Can you work these out from the model? Positions are in its coordinate system, mm. Give positions to 0.01 mm unless a question says otherwise; leave off trailing zeros. Write each loop counter-clockwise with the first axis right and the second up, starting at its lowest first coordinate (ties: lowest second). Pieces come first, ordered by that corner, then holes.
1. Suppose I cut it at C-C (z = 28). Please give me the cut outline in (x, y), and give its area (3 significant figures).
2. Suppose I cut it at D-D (y = -25). Please give me the cut outline in (x, z).
3. Suppose I cut it at B-B (x = 6). Please give me the cut outline in (y, z), and give its area (3 significant figures).
4. Suppose I cut it at A-A (y = 0). Please give me the cut outline in (x, z), and give its area (3 significant figures).
5. I'm going to push a flat-ended pin straight in: pin 1 (5 mm diameter, centred on x = 6, y = 25, fed in from -Z). Where does the tip first touch, or does it pass through?
6. If I drill on probe 1 along Y at (x, z) = (5.25, -16), over which ranges is the centre line in solid material (lowest first)?
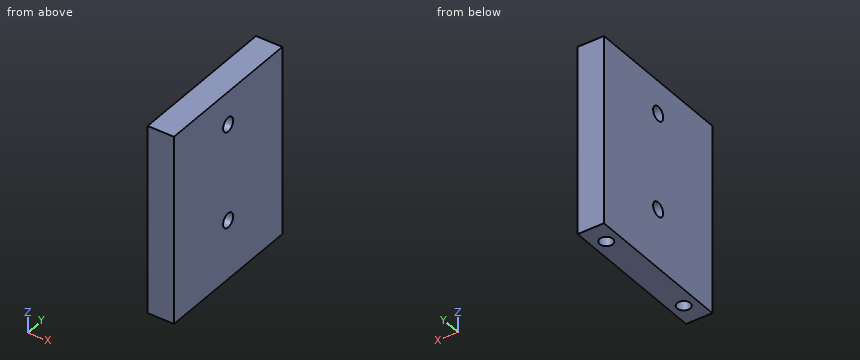
Autodesk Inventor part; units mm, degrees
ref_plane "YZ Plane" through (0, 0, 0) normal (1, 0, 0) x (0, 1, 0)
ref_plane "XZ Plane" through (0, 0, 0) normal (0, 1, 0) x (-1, 0, 0)
ref_plane "XY Plane" through (0, 0, 0) normal (0, 0, 1) x (1, 0, 0)
sketch "Sketch1" plane through (0, 0, 0) normal (1, 0, 0) x (0, 1, 0)
  line L0 (-35, 43) -> (35, 43)
  line L1 (35, 43) -> (35, -43)
  line L2 (35, -43) -> (-35, -43)
  line L3 (-35, -43) -> (-35, 43)
  line L4 (-35, 43) -> (35, -43) construction
  line L5 (35, 43) -> (-35, -43) construction
  point P0 (0, 0)
  dimension "d0" = 86
  dimension "d1" = 70
extrude "Extrusion1" add sketch "Sketch1" along normal blind 12
ref_plane "Work Plane1" through (0, 0, 43) normal (0, 1, 0) x (1, 0, 0)
sketch "Sketch2" plane through (0, -35, -43) normal (0, 0, -1) x (-1, 0, 0)
  circle A0 centre (-6, 60) radius 3
  circle A1 centre (-6, 35) radius 3 construction
  circle A2 centre (-6, 10) radius 3
  line L0 (0, 70) -> (-12, 70)
  line L1 (-6, 70) -> (-6, 0) construction
  line L2 (0, 0) -> (-12, 0)
  point P0 (0, 35)
  dimension "d4" = 6
  dimension "d5" = 25
  dimension "d6" = 25
extrude "Extrusion2" cut sketch "Sketch2" against normal blind 15
sketch "Sketch3" plane through (12, 0, 0) normal (1, 0, 0) x (0, 0, -1)
  circle A0 centre (-46.1752, 0) radius 3
  circle A1 centre (-111.1482, 0) radius 3
  circle A2 centre (-90.1752, 0) radius 3
  point P0 (0, 0)
extrude "Extrusion3" cut sketch "Sketch3" against normal through all
sketch "Sketch4" plane through (0, 0, 0) normal (-1, 0, 0) x (0, 0, 1)
  circle A0 centre (28, 0) radius 3 construction
  circle A1 centre (-16, 0) radius 3 construction
  circle A2 centre (28, 0) radius 3.25
  circle A3 centre (-16, 0) radius 3.25
  point P0 (0, 0)
  dimension "d13" = 0.25
  dimension "d14" = 0.25
extrude "Extrusion4" cut sketch "Sketch4" against normal through all
thread "Thread1"
thread "Thread2"
properties part number "MotorHolderLongAxisBottom"
Checks:
1. outline: (0, -35) - (12, -35) - (12, -3.25) - (0, -3.25) - close; (0, 3.25) - (12, 3.25) - (12, 35) - (0, 35) - close
1. area: 762 mm2
2. outline: (0, -43) - (3, -43) - (3, -28) - (9, -28) - (9, -43) - (12, -43) - (12, 43) - (0, 43) - close
3. outline: (-35, -43) - (-28, -43) - (-28, -28) - (-22, -28) - (-22, -43) - (22, -43) - (22, -28) - (28, -28) - (28, -43) - (35, -43) - (35, 43) - (-35, 43) - close; hole circle Ø6.5 at (0, -16); hole circle Ø6.5 at (0, 28)
3. area: 5,770 mm2
4. outline: (0, -43) - (12, -43) - (12, -19.25) - (0, -19.25) - close; (0, -12.75) - (12, -12.75) - (12, 24.75) - (0, 24.75) - close; (0, 31.25) - (12, 31.25) - (12, 43) - (0, 43) - close
4. area: 876 mm2
5. pin 1: stops at z = -28
6. probe 1: y = -35 to -3.25, 3.25 to 35
